Part model, mm, in its own coordinate system. A direction names the side the tool comes from. Round coordinates to 2 decimals unless told otherwise and drop trailing zeros. Write each loop counter-clockwise with the first axis right and the second up, starting at its lowest first coordinate (ties: lowest second). Pieces come first, ordered by that corner, then holes. Notation, with made-up numbers: M 3.5,-13 L 11.5,-13 A3 ccw 11.5,-8 Z; hole C 89.25,88 d1. An arc over 180 degrees is marked long. Use one line per item in the form item = value. Start each with the question number.
Item 1: Cut at C-C, the plane x = -9.5. Give the cut face in (y, z), then the cut area to 3 significant figures.
Item 2: Which spindle directions (+Z, -Z, +X, -X, +Y, -Y) get a long thin tool onto all of the face, cutting with end or side? Do faces 1 (the face through (-21, -147.5, -27)), 2 (the face through (0, -145, -13.25)), 3 (the face through (17, -153, -47)), 4 (the face through (-23, -28, -16.25)). Say none if no direction does.
Item 3: Probe L1, parallel to Z at x = -20.15, y = -12.75; L2, parallel to Z at x = -20.25, y = -135.75; L3, parallel to X at y = -86, z = -12. List the from-to ranges inside material, lowest first.
Item 4: Cut at B-B, the plane y = -141.5. Give the cut face in (x, z).
Item 5: Cut at A-A, the plane y = -50. Give the cut face in (x, z).
Item 6: Cut at D-D, the plane y = -92. Give the cut face in (x, z).
Item 7: Flat gauge pins, fed straight in: pin 1 Ø1.5 at (x, z) = (15.5, -35.5) entering from +Y; pin 2 Ø3 at (x, y) = (22.5, -30.5) entering from -Z; pin 3 Ø4 at (x, z) = (1, -47.5) entering from -Y. Where does each tip first touch, or does it go through?
Item 8: Mould opens along Z. For faces 5 (the face through (17, -140, -28)), 6 (the face through (23.03, -46.89, -4.63)), 7 (the face through (-21.96, -13.67, -31.65)), 8 (the face through (23.03, -46.63, -50.11)) say: +Z half, -Z half, draft (parallel to the pull), parting line (faces both ways), or undercut.
from build123d import *

# Parameters (mm, degrees)
SKETCH1_W           = 50
SKETCH1_H           = 170
BOSS_EXTRUDE1_DEPTH = 55
SKETCH2_W           = 34
SKETCH2_H           = 27
CUT_EXTRUDE1_DEPTH  = 181.416185527
SKETCH3_W           = 10
SKETCH3_H           = 24
SKETCH3_R           = 4.25
SKETCH3_R_2         = 1
CUT_EXTRUDE2_DEPTH  = 186.539753153
SKETCH4_W           = 2
SKETCH4_H           = 24
CUT_EXTRUDE3_DEPTH  = 178.623196683
SKETCH5_W           = 6.25
SKETCH5_H           = 11.25
CUT_EXTRUDE4_DEPTH  = 186.539753153
SKETCH6_W           = 38
SKETCH6_H           = 10
CUT_EXTRUDE5_DEPTH  = 181.416185527
SKETCH8_W           = 13.25
SKETCH8_H           = 2.25
CUT_EXTRUDE7_DEPTH  = 186.539753153
SKETCH9_W           = 34
SKETCH9_H           = 35.25
CUT_EXTRUDE8_DEPTH  = 179.297679458
SKETCH11_W          = 13.25
SKETCH11_H          = 20.25
CUT_EXTRUDE9_DEPTH  = 184.480414486
SKETCH12_W          = 28.5
SKETCH12_H          = 15
BOSS_EXTRUDE2_DEPTH = 8
SKETCH14_W          = 34
SKETCH14_H          = 15
SKETCH14_H_2        = 10.25
BOSS_EXTRUDE3_DEPTH = 13.25
SKETCH16_R          = 4.5
SKETCH16_R_2        = 2.5
CUT_EXTRUDE13_DEPTH = 8
SKETCH17_W          = 16.25
SKETCH17_H          = 18
CUT_EXTRUDE14_DEPTH = 175.384811552
CUT_EXTRUDE15_DEPTH = 175.384811552
SKETCH20_W          = 42
SKETCH20_H          = 6.25
SKETCH20_H_2        = 18
SKETCH20_H_3        = 58.75
CUT_EXTRUDE18_DEPTH = 169.923244404
SKETCH22_R          = 4.5
SKETCH22_R_2        = 1.45
BOSS_EXTRUDE4_DEPTH = 8
SKETCH23_W          = 2
SKETCH23_H          = 10
CUT_EXTRUDE19_DEPTH = 165.352137193
FILLET1_R           = 10


with BuildPart() as part:
    # Sketch1 → Boss-Extrude1 (new body)
    with BuildSketch(Plane.XY):
        with Locations((0, -85)):
            Rectangle(SKETCH1_W, SKETCH1_H)
    extrude(amount=-BOSS_EXTRUDE1_DEPTH)

    # Sketch2 → Cut-Extrude1 (cut, through all)
    with BuildSketch(Plane.XY):
        with Locations((0, -13.5)):
            Rectangle(SKETCH2_W, SKETCH2_H)
    extrude(amount=-CUT_EXTRUDE1_DEPTH, mode=Mode.SUBTRACT)

    # Sketch3 → Cut-Extrude2 (cut, through all)
    with BuildSketch(Plane(origin=(25, 0, 0), x_dir=(0, 0, -1), z_dir=(1, 0, 0))):
        with Locations((50, -12)):
            Rectangle(SKETCH3_W, SKETCH3_H)
        with Locations((5, -12)):
            Rectangle(SKETCH3_W, SKETCH3_H)
        with Locations(Location((27.5, -12.75, 0), (0, 0, 90))):
            Circle(SKETCH3_R)
        with Locations(Location((35.5, -12.75, 0), (0, 0, 90))):
            Circle(SKETCH3_R_2)
        with Locations(Location((27.5, -4.75, 0), (0, 0, 90))):
            Circle(SKETCH3_R_2)
        with Locations(Location((27.5, -20.75, 0), (0, 0, 90))):
            Circle(SKETCH3_R_2)
        with Locations(Location((19.5, -12.75, 0), (0, 0, 90))):
            Circle(SKETCH3_R_2)
    extrude(amount=-CUT_EXTRUDE2_DEPTH, mode=Mode.SUBTRACT)

    # Sketch4 → Cut-Extrude3 (cut, through all)
    with BuildSketch(Plane.XY.offset(-10)):
        with Locations((-18, -12)):
            Rectangle(SKETCH4_W, SKETCH4_H)
        with Locations((18, -12)):
            Rectangle(SKETCH4_W, SKETCH4_H)
    extrude(amount=-CUT_EXTRUDE3_DEPTH, mode=Mode.SUBTRACT)

    # Sketch5 → Cut-Extrude4 (cut, through all)
    with BuildSketch(Plane(origin=(25, 0, 0), x_dir=(0, 0, -1), z_dir=(1, 0, 0))):
        with BuildLine():
            Line((45, 0), (10, 0))
            Line((10, 0), (10, -12.75))
            Line((10, -12.75), (16.25, -12.75))
            ThreePointArc((16.25, -12.75), (27.5, -1.5), (38.75, -12.75))
            Line((38.75, -12.75), (45, -12.75))
            Line((45, -12.75), (45, 0))
        make_face()
        with Locations((13.125, -18.375)):
            Rectangle(SKETCH5_W, SKETCH5_H)
        with Locations((41.875, -18.375)):
            Rectangle(SKETCH5_W, SKETCH5_H)
    extrude(amount=-CUT_EXTRUDE4_DEPTH, mode=Mode.SUBTRACT)

    # Sketch6 → Cut-Extrude5 (cut, through all)
    with BuildSketch(Plane.XY):
        with Locations((0, -29)):
            Rectangle(SKETCH6_W, SKETCH6_H)
    extrude(amount=-CUT_EXTRUDE5_DEPTH, mode=Mode.SUBTRACT)

    # Sketch8 → Cut-Extrude7 (cut, through all)
    with BuildSketch(Plane(origin=(25, 0, 0), x_dir=(0, 0, -1), z_dir=(1, 0, 0))):
        with BuildLine():
            Line((27.5, -157.5), (27.5, -132.5))
            Line((27.5, -132.5), (13.25, -132.5))
            Line((13.25, -132.5), (13.25, -167.75))
            Line((13.25, -167.75), (17.25, -167.75))
            ThreePointArc((17.25, -167.75), (20.252155493, -160.502155493), (27.5, -157.5))
        make_face()
        with BuildLine():
            Line((41.75, -167.75), (41.75, -132.5))
            Line((41.75, -132.5), (27.5, -132.5))
            Line((27.5, -132.5), (27.5, -157.5))
            ThreePointArc((27.5, -157.5), (34.747844507, -160.502155493), (37.75, -167.75))
            Line((37.75, -167.75), (41.75, -167.75))
        make_face()
        with Locations((48.375, -168.875)):
            Rectangle(SKETCH8_W, SKETCH8_H)
        with Locations((6.625, -168.875)):
            Rectangle(SKETCH8_W, SKETCH8_H)
        with BuildLine():
            Line((17.25, -167.75), (13.25, -167.75))
            Line((13.25, -167.75), (13.25, -170))
            Line((13.25, -170), (17.5, -170))
            ThreePointArc((17.5, -170), (17.31269172, -168.881923142), (17.25, -167.75))
        make_face()
        with BuildLine():
            Line((41.75, -170), (41.75, -167.75))
            Line((41.75, -167.75), (37.75, -167.75))
            ThreePointArc((37.75, -167.75), (37.68730828, -168.881923142), (37.5, -170))
            Line((37.5, -170), (41.75, -170))
        make_face()
        with BuildLine():
            Line((27.5, -167.75), (27.5, -157.5))
            ThreePointArc((27.5, -157.5), (20.252155493, -160.502155493), (17.25, -167.75))
            Line((17.25, -167.75), (27.5, -167.75))
        make_face()
        with BuildLine():
            ThreePointArc((37.75, -167.75), (34.747844507, -160.502155493), (27.5, -157.5))
            Line((27.5, -157.5), (27.5, -167.75))
            Line((27.5, -167.75), (37.75, -167.75))
        make_face()
        with BuildLine():
            Line((27.5, -170), (27.5, -167.75))
            Line((27.5, -167.75), (17.25, -167.75))
            ThreePointArc((17.25, -167.75), (17.31269172, -168.881923142), (17.5, -170))
            Line((17.5, -170), (27.5, -170))
        make_face()
        with BuildLine():
            ThreePointArc((37.5, -170), (37.68730828, -168.881923142), (37.75, -167.75))
            Line((37.75, -167.75), (27.5, -167.75))
            Line((27.5, -167.75), (27.5, -170))
            Line((27.5, -170), (37.5, -170))
        make_face()
    extrude(amount=-CUT_EXTRUDE7_DEPTH, mode=Mode.SUBTRACT)

    # Sketch9 → Cut-Extrude8 (cut, through all)
    with BuildSketch(Plane.XY):
        with Locations((0, -150.125)):
            Rectangle(SKETCH9_W, SKETCH9_H)
    extrude(amount=-CUT_EXTRUDE8_DEPTH, mode=Mode.SUBTRACT)

    # Sketch11 → Cut-Extrude9 (cut, through all)
    with BuildSketch(Plane(origin=(25, 0, 0), x_dir=(0, 0, -1), z_dir=(1, 0, 0))):
        with BuildLine():
            ThreePointArc((17.25, -167.75), (20.252155493, -160.502155493), (27.5, -157.5))
            Line((27.5, -157.5), (27.5, -147.5))
            Line((27.5, -147.5), (13.25, -147.5))
            Line((13.25, -147.5), (13.25, -167.75))
            Line((13.25, -167.75), (17.25, -167.75))
        make_face()
        with BuildLine():
            Line((27.5, -147.5), (27.5, -157.5))
            ThreePointArc((27.5, -157.5), (34.747844507, -160.502155493), (37.75, -167.75))
            Line((37.75, -167.75), (41.75, -167.75))
            Line((41.75, -167.75), (41.75, -147.5))
            Line((41.75, -147.5), (27.5, -147.5))
        make_face()
        with Locations((48.375, -157.625)):
            Rectangle(SKETCH11_W, SKETCH11_H)
        with Locations((6.625, -157.625)):
            Rectangle(SKETCH11_W, SKETCH11_H)
    extrude(amount=-CUT_EXTRUDE9_DEPTH, mode=Mode.SUBTRACT)

    # Sketch12 → Boss-Extrude2 (add)
    with BuildSketch(Plane(origin=(25, 0, 0), x_dir=(0, 0, -1), z_dir=(1, 0, 0))):
        with Locations((27.5, -140)):
            Rectangle(SKETCH12_W, SKETCH12_H)
    boss_extrude2 = extrude(amount=-BOSS_EXTRUDE2_DEPTH)

    # Mirror1: Boss-Extrude2 across plane
    add(boss_extrude2.mirror(Plane(origin=(0, 0, 0), x_dir=(0, 0, 1), z_dir=(1, 0, 0))))

    # Sketch14 → Boss-Extrude3 (add)
    with BuildSketch(Plane.XY):
        with Locations((0, -140)):
            Rectangle(SKETCH14_W, SKETCH14_H)
        with Locations((0, -152.625)):
            Rectangle(SKETCH14_W, SKETCH14_H_2)
    boss_extrude3 = extrude(amount=-BOSS_EXTRUDE3_DEPTH)

    # Mirror2: Boss-Extrude3 across plane
    add(boss_extrude3.mirror(Plane.XY.offset(-27.5)))

    # Sketch16 → Cut-Extrude13 (cut)
    # profile 1 of 3: a face of its own
    with BuildSketch(Plane(origin=(25, 0, 0), x_dir=(0, 0, -1), z_dir=(1, 0, 0))):
        with Locations(Location((16.5, -135.75, 0), (0, 0, 90))):
            Circle(SKETCH16_R)
        with Locations((16.5, -135.75)):
            Circle(SKETCH16_R_2, mode=Mode.SUBTRACT)
    # profile 2 of 3: a face of its own
    with BuildSketch(Plane(origin=(25, 0, 0), x_dir=(0, 0, -1), z_dir=(1, 0, 0))):
        with Locations((16.5, -135.75)):
            Circle(SKETCH16_R_2)
    # profile 3 of 3: a face of its own
    with BuildSketch(Plane(origin=(25, 0, 0), x_dir=(0, 0, -1), z_dir=(1, 0, 0))):
        with Locations(Location((38.5, -135.75, 0), (0, 0, 90))):
            Circle(SKETCH16_R)
    cut_extrude13 = extrude(amount=-CUT_EXTRUDE13_DEPTH, mode=Mode.SUBTRACT)

    # Mirror3: Cut-Extrude13 across plane
    add(cut_extrude13.mirror(Plane(origin=(0, 0, 0), x_dir=(0, 0, 1), z_dir=(1, 0, 0))), mode=Mode.SUBTRACT)

    # Sketch17 → Cut-Extrude14 (cut, through all)
    with BuildSketch(Plane(origin=(25, 0, 0), x_dir=(0, 0, -1), z_dir=(1, 0, 0))):
        with Locations((46.875, -33)):
            Rectangle(SKETCH17_W, SKETCH17_H)
        with Locations((8.125, -33)):
            Rectangle(SKETCH17_W, SKETCH17_H)
    extrude(amount=-CUT_EXTRUDE14_DEPTH, mode=Mode.SUBTRACT)

    # Sketch18 → Cut-Extrude15 (cut, through all)
    with BuildSketch(Plane(origin=(25, 0, 0), x_dir=(0, 0, -1), z_dir=(1, 0, 0))):
        with BuildLine():
            ThreePointArc((0, -58.25), (4.759514806, -46.759514806), (16.25, -42))
            Line((16.25, -42), (0, -42))
            Line((0, -42), (0, -58.25))
        make_face()
        with BuildLine():
            Line((55, -42), (38.75, -42))
            ThreePointArc((38.75, -42), (50.240485194, -46.759514806), (55, -58.25))
            Line((55, -58.25), (55, -42))
        make_face()
    extrude(amount=-CUT_EXTRUDE15_DEPTH, mode=Mode.SUBTRACT)

    # Sketch20 → Cut-Extrude18 (cut, through all)
    with BuildSketch(Plane(origin=(0, 0, -55), x_dir=(-1, 0, 0), z_dir=(0, 0, -1))):
        with Locations((0, -55.125)):
            Rectangle(SKETCH20_W, SKETCH20_H)
        with Locations((0, -43)):
            Rectangle(SKETCH20_W, SKETCH20_H_2)
        with Locations((0, -87.625)):
            Rectangle(SKETCH20_W, SKETCH20_H_3)
    extrude(amount=-CUT_EXTRUDE18_DEPTH, mode=Mode.SUBTRACT)

    # Sketch22 → Boss-Extrude4 (add)
    # profile 1 of 2: a face of its own
    with BuildSketch(Plane.ZY.offset(25)):
        with Locations(Location((-38.5, -135.75, 0), (0, 0, 90))):
            Circle(SKETCH22_R)
        with Locations(Location((-38.5, -135.75, 0), (0, 0, 270))):
            Circle(SKETCH22_R_2, mode=Mode.SUBTRACT)
    # profile 2 of 2: a face of its own
    with BuildSketch(Plane.ZY.offset(25)):
        with Locations(Location((-16.5, -135.75, 0), (0, 0, 90))):
            Circle(SKETCH22_R)
        with Locations(Location((-16.5, -135.75, 0), (0, 0, 270))):
            Circle(SKETCH22_R_2, mode=Mode.SUBTRACT)
    boss_extrude4 = extrude(amount=-BOSS_EXTRUDE4_DEPTH)

    # Mirror4: Boss-Extrude4 across plane
    add(boss_extrude4.mirror(Plane(origin=(0, 0, 0), x_dir=(0, 0, 1), z_dir=(1, 0, 0))))

    # Sketch23 → Cut-Extrude19 (cut, through all)
    with BuildSketch(Plane(origin=(0, 0, -38.75), x_dir=(-1, 0, 0), z_dir=(0, 0, -1))):
        with Locations((-20, -29)):
            Rectangle(SKETCH23_W, SKETCH23_H)
        with Locations((20, -29)):
            Rectangle(SKETCH23_W, SKETCH23_H)
    extrude(amount=-CUT_EXTRUDE19_DEPTH, mode=Mode.SUBTRACT)

    # Fillet1
    fillet1_edges = [part.edges().sort_by_distance(p)[0] for p in [
        (0, -157.75, 0),
        (0, -157.75, -55),
    ]]
    fillet(fillet1_edges, radius=FILLET1_R)


solid = part.part
Model answer:
q1.outline = M -157.75,-45 A10 ccw -147.75,-55 L -117,-55 L -117,0 L -147.75,0 A10 ccw -157.75,-10 L -157.75,-13.25 L -132.5,-13.25 L -132.5,-41.75 L -157.75,-41.75 Z
q1.area = 1,480 mm²
q2.face_1 = +Z, -Z, -X, -Y
q2.face_2 = -Y
q2.face_3 = +Z, -Z, +X, -Y
q2.face_4 = +Z, +X, -X, +Y
q3.L1 = -38.75 to -36.5, -34.5 to -31.75, -23.25 to -20.5, -18.5 to -16.25
q3.L2 = -55 to -39.95, -37.05 to -17.95, -15.05 to 0
q3.L3 = -25 to -21, 21 to 25
q4.outline = M -25,-55 L 25,-55 L 25,0 L -25,0 Z; hole M -17,-41.75 L 17,-41.75 L 17,-13.25 L -17,-13.25 Z
q5.outline = M -25,-52.75 L -21,-52.75 L -21,-2.25 L -25,-2.25 Z; M 21,-52.75 L 25,-52.75 L 25,-2.25 L 21,-2.25 Z
q6.outline = M -25,-55 L -21,-55 L -21,0 L -25,0 Z; M 21,-55 L 25,-55 L 25,0 L 21,0 Z
q7.pin_1 = -117
q7.pin_2 = -38.75
q7.pin_3 = -157.74
q8.face_5 = undercut
q8.face_6 = +Z half
q8.face_7 = undercut
q8.face_8 = -Z half
